Autodesk Inventor part; units mm, degrees
ref_plane "YZ Plane" through (0, 0, 0) normal (1, 0, 0) x (0, 1, 0)
ref_plane "XZ Plane" through (0, 0, 0) normal (0, 1, 0) x (-1, 0, 0)
ref_plane "XY Plane" through (0, 0, 0) normal (0, 0, 1) x (1, 0, 0)
sketch "Sketch1" plane through (0, 0, 0) normal (1, 0, 0) x (0, 1, 0)
  circle A0 centre (0, 1.3072) radius 101.6
  circle A1 centre (0, 1.3072) radius 107.95
  point P0 (0, 0)
  dimension "d0" = 203.2
  dimension "d1" = 215.9
extrude "Extrusion1" add sketch "Sketch1" along normal blind 50.8
sketch "Sketch2" plane through (50.8, 0, 1.3072) normal (1, 0, 0) x (0, 0, -1)
  circle A0 centre (0, 0) radius 101.6
  circle A1 centre (0, 0) radius 107.95
  line L0 (127, 0) -> (127, 127)
  line L1 (127, 127) -> (0, 127)
  line L2 (0, 127) -> (0, 107.95)
  arc A2 (107.95, 0) -> (0, 107.95) centre (0, 0) ccw
  line L3 (107.95, 0) -> (127, 0)
  dimension "d13" = 127
  dimension "d15" = 127
extrude "Extrusion2" add sketch "Sketch2" against normal blind 50.8 contours A1 L2 L1 L0 L3
sketch "Sketch3" plane through (50.8, 0, 0) normal (1, 0, 0) x (0, 0, -1)
  line L0 (-164.0903, 142.5246) -> (-1.3072, 142.5246)
  line L1 (-20.2178, -157.5435) -> (-164.0903, -157.5435)
  line L2 (-164.0903, -157.5435) -> (-164.0903, 142.5246)
  line L3 (195.7449, 0) -> (-1.3072, 0)
  line L4 (-20.2178, -149.5335) -> (195.7449, -149.5335)
  line L5 (195.7449, -149.5335) -> (195.7449, 0)
  line L6 (106.6428, 0) -> (125.6928, 0)
  line L7 (-1.3072, 142.5246) -> (-1.3072, 0)
  line L8 (-20.2178, -149.5335) -> (-20.2178, -157.5435)
  line L9 (-1.3072, 127) -> (-1.3072, 107.95)
  point P0 (0, 0)
  dimension "d18" = 0
  dimension "d19" = 0
extrude "Extrusion3" cut sketch "Sketch3" against normal blind 50.8
properties part number "Ramp"
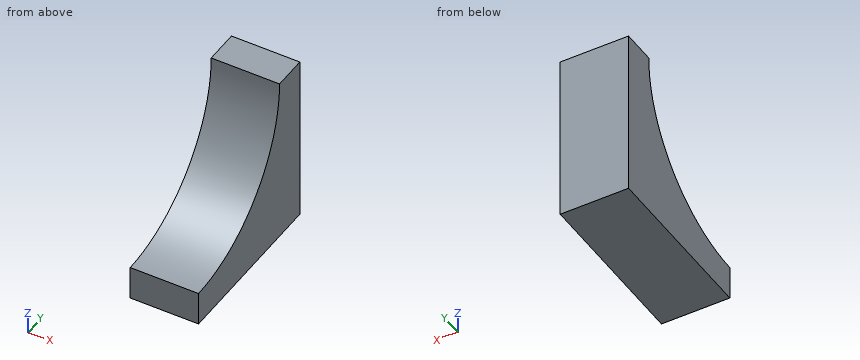
The listing builds one solid part. Answer for the finished solid, in the listing's coordinates (mm). Give positions to 0.01 mm unless a question says otherwise; leave off trailing zeros. Write each loop counter-clockwise with the first axis right and the second up, starting at its lowest first coordinate (ties: lowest second). Pieces come first, ordered by that corner, then holes. Notation, with made-up numbers: M 22,53 L 27,53 A22 cw 27,61 Z; hole C -34.5,80 d11. An arc over 180 degrees is marked long. Write each question's results on one line, items separated by ' | '.
Q1. Consider L1, parallel to Y at x = 9, z = -88; L2, parallel to Z at x = 37, y = 75; L3, parallel to Y at x = 25, z = -44. Determine where each line is inside the solid, lowest interval first. Write a range as from..to.
Output values:
L1: 48.44..127 | L2: -125.69..-67.23 | L3: 90.94..127
Q2. Section C-C, the plane y = 34 is taken. Write down the section's boundary in (x, z).
Output values:
outline: M 0,-125.69 L 50.8,-125.69 L 50.8,-94.43 L 0,-94.43 Z
Q3. Section B-B, the plane z = -86.5 is taken. Write down the section's boundary in (x, y).
Output values:
outline: M 0,51.11 L 50.8,51.11 L 50.8,127 L 0,127 Z
Q4. Flat-ended cylindrical pins translate along their axes: P1, Ø5, axis at x = 12.5, y = 53.5, coming from the +Z side; P2, Ø1, axis at x = 5.5, y = 92.5, coming from the +Z side; P3, Ø2, axis at x = 30, z = -43.5, coming from the -Y side. Find the tip coordinate at first contact, or state that the pin passes through.
Output values:
P1: z = -83.47 | P2: z = -39.6 | P3: y = 90.69
Q5. Section A-A, the plane x = 17 is taken. Write down the section's boundary in (y, z), then the cut area to 3 significant figures.
Output values:
outline: M 0,-125.69 L 127,-125.69 L 127,1.31 L 101.6,1.31 A101.6 cw 0,-100.29 Z | area: 8,020 mm2
